CAD build for the part. Positions are in the model's coordinates, mm. Face numbers are marked on the shaded views. A direction names the side the tool comes from. Give positions to 0.01 mm unless a question says otherwise; leave off trailing zeros. Loops run counter-clockwise (first coordinate to the right, second up) from the corner with the lowest first, then second, coordinate; pieces in that order, holes last.
Item 1: Saw through at C-C on z = -29.5. Give the cut face in (x, y), plus the area to 3 significant figures.
Item 2: Probe probe 1 along Y at (x, z) = (0, -37.2); probe 2 along Z at (x, y) = (6.75, 8.5); probe 3 along Y at (x, z) = (0, 10.15). List the from-to ranges inside material, lowest first.
Item 3: Which spindle directions (+Z, -Z, +X, -X, +Y, -Y) get a long thin tool onto all of the face, cutting with end or side? Do the marked faces 1, 2 and 3. Say none if no direction does.
Item 4: Saw through at A-A on x = 0. Give the number of separate pieces and of enclosed holes in the cut face, plus the area to 3 significant figures.
Item 5: Drop flat-ended pins along their axis: P1, Ø1, axis at y = -6.5, z = 6.5, coming from the +X side; P2, Ø1.5, axis at x = 2, z = 5, coming from the -Y side; P3, Ø2, axis at x = 8, z = -0.5, coming from the -Y side. Give the stop position or say it passes through.
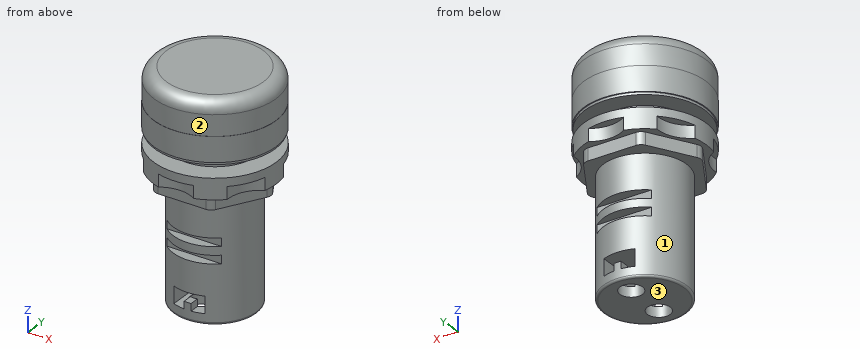
from build123d import *

# Parameters (mm, degrees)
ESBO_O1_R             = 14.75
EXTRUS_O1_DEPTH       = 6
ESBO_O2_R             = 10
EXTRUS_O2_DEPTH       = 40
ESBO_O3_R             = 11
EXTRUS_O3_DEPTH       = 5
ESBO_O4_R             = 14.7
ESBO_O4_R_2           = 12.5
EXTRUS_O4_DEPTH       = 8
EXTRUS_O5_START       = -2
ESBO_O5_R             = 14.7
EXTRUS_O5_DEPTH       = 2
FILETE2_R             = 3
ESBO_O6_R             = 14.5
EXTRUS_O6_DEPTH       = 0.6
EXTRUS_O7_START       = 8
ESBO_O7_R             = 14.75
EXTRUS_O7_DEPTH       = 5
CORTE_EXTRUS_O1_DEPTH = 3
CIRPATTERN1_COUNT     = 6
EXTRUS_O8_DEPTH       = 3
FILETE3_R             = 0.5
CORTE_EXTRUS_O2_START = -14
ESBO_O10_W            = 40
ESBO_O10_H            = 25
ESBO_O10_W_2          = 30
ESBO_O10_H_2          = 15
CORTE_EXTRUS_O2_DEPTH = 2
LPATTERN1_COUNT       = 2
LPATTERN1_PITCH       = 4
ESBO_O11_R            = 2.75
CORTE_EXTRUS_O3_DEPTH = 5
CORTE_EXTRUS_O4_DEPTH = 12.5


with BuildPart() as part:
    # Esboço1 → Extrusão1 (new body)
    with BuildSketch(Plane.XY):
        Circle(ESBO_O1_R)
    extrude(amount=EXTRUS_O1_DEPTH)

    # Esboço2 → Extrusão2 (add)
    with BuildSketch(Plane(origin=(0, 0, 0), x_dir=(-1, 0, 0), z_dir=(0, 0, -1))):
        with Locations(Location((0, 0, 0), (0, 0, 180))):
            Circle(ESBO_O2_R)
    extrude(amount=EXTRUS_O2_DEPTH)

    # Esboço3 → Extrusão3 (add)
    with BuildSketch(Plane.XY.offset(6)):
        Circle(ESBO_O3_R)
    extrude(amount=EXTRUS_O3_DEPTH)

    # Esboço4 → Extrusão4 (add)
    with BuildSketch(Plane.XY.offset(6)):
        Circle(ESBO_O4_R)
        Circle(ESBO_O4_R_2, mode=Mode.SUBTRACT)
    extrude(amount=EXTRUS_O4_DEPTH)

    # Esboço5 → Extrusão5 (add)
    with BuildSketch(Plane.XY.offset(14).offset(EXTRUS_O5_START)):
        Circle(ESBO_O5_R)
    extrude(amount=EXTRUS_O5_DEPTH)

    # Filete2
    filete2_edges = [part.edges().sort_by_distance(p)[0] for p in [
        (-14.7, 0, 14),
    ]]
    fillet(filete2_edges, radius=FILETE2_R)

    # Esboço6 → Extrusão6 (add)
    with BuildSketch(Plane(origin=(0, 0, 0), x_dir=(-1, 0, 0), z_dir=(0, 0, -1))):
        with Locations(Location((0, 0, 0), (0, 0, 180))):
            Circle(ESBO_O6_R)
    extrude(amount=EXTRUS_O6_DEPTH)

    # Esboço7 → Extrusão7 (add)
    with BuildSketch(Plane(origin=(0, 0, -0.6), x_dir=(-1, 0, 0), z_dir=(0, 0, -1)).offset(EXTRUS_O7_START)):
        with Locations(Location((0, 0, 0), (0, 0, 180))):
            Circle(ESBO_O7_R)
    extrude(amount=-EXTRUS_O7_DEPTH)

    # Esboço8 → Corte-extrusão1 (cut)
    with BuildSketch(Plane(origin=(0, 0, -8.6), x_dir=(-1, 0, 0), z_dir=(0, 0, -1))):
        with BuildLine():
            ThreePointArc((-4.25, 14.124446892), (0, 12.843637989), (4.25, 14.124446892))
            ThreePointArc((4.25, 14.124446892), (0, 15.884854532), (-4.25, 14.124446892))
        make_face()
    corte_extrus_o1 = extrude(amount=-CORTE_EXTRUS_O1_DEPTH, mode=Mode.SUBTRACT)

    # CirPattern1: Corte-extrusão1 ×6 about axis
    cirpattern1_axis = Axis((0, 0, 0), (0, 0, 1))
    for i in range(1, CIRPATTERN1_COUNT):
        add(corte_extrus_o1.rotate(cirpattern1_axis, i * 360 / CIRPATTERN1_COUNT), mode=Mode.SUBTRACT)

    # Esboço9 → Extrusão8 (add)
    with BuildSketch(Plane(origin=(0, 0, -8.6), x_dir=(-1, 0, 0), z_dir=(0, 0, -1))):
        with BuildLine():
            Line((-7.505553499, 11), (-13.279056191, 1))
            ThreePointArc((-13.279056191, 1), (-13.547005384, 0), (-13.279056191, -1))
            Line((-13.279056191, -1), (-7.505553499, -11))
            ThreePointArc((-7.505553499, -11), (-6.773502692, -11.732050808), (-5.773502692, -12))
            Line((-5.773502692, -12), (5.773502692, -12))
            ThreePointArc((5.773502692, -12), (6.773502692, -11.732050808), (7.505553499, -11))
            Line((7.505553499, -11), (13.279056191, -1))
            ThreePointArc((13.279056191, -1), (13.547005384, 0), (13.279056191, 1))
            Line((13.279056191, 1), (7.505553499, 11))
            ThreePointArc((7.505553499, 11), (6.773502692, 11.732050808), (5.773502692, 12))
            Line((5.773502692, 12), (-5.773502692, 12))
            ThreePointArc((-5.773502692, 12), (-6.773502692, 11.732050808), (-7.505553499, 11))
        make_face()
    extrude(amount=EXTRUS_O8_DEPTH)

    # Filete3
    filete3_edges = [part.edges().sort_by_distance(p)[0] for p in [
        (-10, 0, -40),
    ]]
    fillet(filete3_edges, radius=FILETE3_R)

    # Esboço10 → Corte-extrusão2 (cut)
    with BuildSketch(Plane(origin=(0, 0, -40), x_dir=(-1, 0, 0), z_dir=(0, 0, -1)).offset(CORTE_EXTRUS_O2_START)):
        Rectangle(ESBO_O10_W, ESBO_O10_H)
        Rectangle(ESBO_O10_W_2, ESBO_O10_H_2, mode=Mode.SUBTRACT)
    corte_extrus_o2 = extrude(amount=-CORTE_EXTRUS_O2_DEPTH, mode=Mode.SUBTRACT)

    # LPattern1: Corte-extrusão2 ×2
    with Locations(*[(0, 0, i * LPATTERN1_PITCH) for i in range(1, LPATTERN1_COUNT)]):
        add(corte_extrus_o2, mode=Mode.SUBTRACT)

    # Esboço11 → Corte-extrusão3 (cut)
    with BuildSketch(Plane(origin=(0, 0, -40), x_dir=(-1, 0, 0), z_dir=(0, 0, -1))):
        with Locations((0, 5)):
            Circle(ESBO_O11_R)
        with Locations(Location((0, -5, 0), (0, 0, 180))):
            Circle(ESBO_O11_R)
    extrude(amount=-CORTE_EXTRUS_O3_DEPTH, mode=Mode.SUBTRACT)

    # 3DSketch2 → Corte-extrusão4 (cut, symmetric)
    with BuildSketch(Plane(origin=(-3.75, 0, -37.527086784), x_dir=(0.8800460423188995, 0, 0.4748883694078451), z_dir=(0, -1, 0))):
        Polygon((0, 0), (2.571694256, -1.387731588), (3.404519941, 0.155631013), (4.879432804, -0.640257987), (4.046607118, -2.183620587), (6.600345317, -3.561662771), (8.52228138, 0), (1.921937352, 3.56166516), align=None)
    extrude(amount=CORTE_EXTRUS_O4_DEPTH, both=True, mode=Mode.SUBTRACT)


solid = part.part
Results below:
1. outline: circle Ø20 at (0, 0)
1. area: 314 mm2
2. probe 1: y = -10 to -7.75, -2.25 to 2.25, 7.75 to 10
2. probe 2: z = -11.6 to -3.6, -0.6 to 11, 12 to 14
2. probe 3: y = -14.7 to -12.5, -11 to 11, 12.5 to 14.7
3. face 1: -Z
3. face 2: +Z
3. face 3: -Z, +X, -X, +Y, -Y
4. separate pieces: 4
4. enclosed holes: 1
4. area: 1,110 mm2
5. P1: stops at x = 13.42
5. P2: stops at y = -14.7
5. P3: stops at y = -12.91
